The listing builds one solid part. Answer for the finished solid, in the listing's coordinates (mm). A direction names the side the tool comes from. Coordinates: 2 decimals unless noted, no trailing zeros. Loops run counter-clockwise (first coordinate to the right, second up) from the corner with the lowest first, then second, coordinate; pieces in that order, holes last. Notation, with made-up numbers: (48.25, -23.5) - (62.25, -23.5) arc R14 ccw to (62.25, -11.5) - close; hole circle Ø9 at (58, 71.5). An arc over 180 degrees is marked (long way). Write each question's results on one line, items separated by ' | '. Start each with the question number.
(1) Find section B-B on y = 30.5. Determine the outline of the cut face in (x, z).
(2) Determine the mould class of faces 6 (the flat face through (-66, 17, 1)), 7 (the flat face through (-1, 13, -47.5)), 8 (the cylindrical face through (-1.71, 6.75, -32.19)) for opening direction X: released by +X, released by -X, zero draft, split by the parting line, or undercut.
(3) Consider line 1 (X direction, y = 14, z = -22); line 2 (X direction, y = 4.05, z = 0) (3 decimals); line 3 (Z direction, x = 33.5, y = 25). Determine where each line is inside the solid, lowest interval first. Write a range as from..to.
(4) Find section D-D on x = -30. Determine the outline of the cut face in (y, z), then the cut area to 3 significant figures.
(5) Given pin 1 Ø3 at (x, z) = (0, -34.5) entering from +Y; pin 2 Ø3 at (x, z) = (49.5, 2) entering from +Y; pin 3 Ø5.5 at (x, z) = (26.625, 0) entering from +Y, each flat-ended and moving along its own axis, determine where each tip first touches the part or whether it passes through.
(6) For faces 1 (the cylindrical face through (63.5, 24.9, -10.7)), 2 (the flat face through (15, 15, 45)), 3 (the cylindrical face through (-33, 4, -1)), 4 (the flat face through (-10, 20, 28.363)), 5 (the cylindrical face through (-38.535, 1.521, -0.369)), determine the directions among +Z, -Z, +X, -X, +Y, -Y from which every point of the face is accessible in a straight line to the end or side of a thin tool.
(7) Find section C-C on z = -29. Determine the outline of the cut face in (x, y), then the cut area to 3 significant figures.
from build123d import *

# Parameters (mm, degrees)
SKETCH1_W           = 132
SKETCH1_H           = 95
BOSS_EXTRUDE1_DEPTH = 35
SKETCH2_W           = 122
SKETCH2_H           = 85
CUT_EXTRUDE1_DEPTH  = 30
SKETCH4_W           = 5
SKETCH4_H           = 85
BOSS_EXTRUDE2_DEPTH = 30
SKETCH5_R           = 2.5
SKETCH5_R_2         = 1.75
BOSS_EXTRUDE3_DEPTH = 2
FILLET1_R           = 1.5
SKETCH7_W           = 5
SKETCH7_H           = 10
CUT_EXTRUDE3_DEPTH  = 10
SKETCH8_R           = 1.75
SKETCH8_R_2         = 1.7
CUT_EXTRUDE4_DEPTH  = 10
SKETCH9_R           = 4
CUT_EXTRUDE6_DEPTH  = 2
SKETCH11_W          = 5.5
SKETCH11_H          = 12
SKETCH11_H_2        = 10
CUT_EXTRUDE7_DEPTH  = 10
SKETCH13_W          = 5.5
SKETCH13_H          = 10
CUT_EXTRUDE8_DEPTH  = 10
SKETCH14_W          = 5.5
SKETCH14_H          = 12
CUT_EXTRUDE9_DEPTH  = 10
SKETCH15_R          = 1.75
CUT_EXTRUDE10_DEPTH = 10


with BuildPart() as part:
    # Sketch1 → Boss-Extrude1 (new body)
    with BuildSketch(Plane(origin=(0, 0, 0), x_dir=(1, 0, 0), z_dir=(0, 1, 0))):
        Rectangle(SKETCH1_W, SKETCH1_H)
    extrude(amount=BOSS_EXTRUDE1_DEPTH)

    # Sketch2 → Cut-Extrude1 (cut)
    with BuildSketch(Plane(origin=(0, 35, 0), x_dir=(1, 0, 0), z_dir=(0, 1, 0))):
        Rectangle(SKETCH2_W, SKETCH2_H)
    extrude(amount=-CUT_EXTRUDE1_DEPTH, mode=Mode.SUBTRACT)

    # Sketch4 → Boss-Extrude2 (add, through all)
    with BuildSketch(Plane(origin=(0, 5, 0), x_dir=(1, 0, 0), z_dir=(0, 1, 0))):
        with Locations((-10.25, 0)):
            Rectangle(SKETCH4_W, SKETCH4_H)
    extrude(amount=BOSS_EXTRUDE2_DEPTH)

    # Sketch5 → Boss-Extrude3 (add)
    # profile 1 of 4: a face of its own
    with BuildSketch(Plane(origin=(0, 5, 0), x_dir=(1, 0, 0), z_dir=(0, 1, 0))):
        with Locations(Location((55.55, -35.5, 0), (0, 0, 270))):
            Circle(SKETCH5_R)
        with Locations(Location((55.55, -35.5, 0), (0, 0, 270))):
            Circle(SKETCH5_R_2, mode=Mode.SUBTRACT)
    # profile 2 of 4: a face of its own
    with BuildSketch(Plane(origin=(0, 5, 0), x_dir=(1, 0, 0), z_dir=(0, 1, 0))):
        with Locations(Location((-0.75, -35.5, 0), (0, 0, 270))):
            Circle(SKETCH5_R)
        with Locations(Location((-0.75, -35.5, 0), (0, 0, 270))):
            Circle(SKETCH5_R_2, mode=Mode.SUBTRACT)
    # profile 3 of 4: a face of its own
    with BuildSketch(Plane(origin=(0, 5, 0), x_dir=(1, 0, 0), z_dir=(0, 1, 0))):
        with Locations(Location((55.249999996, 34.49935714, 0), (0, 0, 270))):
            Circle(SKETCH5_R)
        with Locations(Location((55.249999996, 34.49935714, 0), (0, 0, 270))):
            Circle(SKETCH5_R_2, mode=Mode.SUBTRACT)
    # profile 4 of 4: a face of its own
    with BuildSketch(Plane(origin=(0, 5, 0), x_dir=(1, 0, 0), z_dir=(0, 1, 0))):
        with Locations(Location((-0.75, 34.5, 0), (0, 0, 270))):
            Circle(SKETCH5_R)
        with Locations(Location((-0.75, 34.5, 0), (0, 0, 270))):
            Circle(SKETCH5_R_2, mode=Mode.SUBTRACT)
    extrude(amount=BOSS_EXTRUDE3_DEPTH)

    # Fillet1
    fillet1_edges = [part.edges().sort_by_distance(p)[0] for p in [
        (55.55, 5, 33),
        (-0.75, 5, 33),
        (55.249999996, 5, -36.99935714),
        (-0.75, 5, -37),
    ]]
    fillet(fillet1_edges, radius=FILLET1_R)

    # Sketch7 → Cut-Extrude3 (cut)
    with BuildSketch(Plane(origin=(-7.75, 0, 0), x_dir=(0, 0, -1), z_dir=(1, 0, 0))):
        with Locations((-25.863290262, 20)):
            Rectangle(SKETCH7_W, SKETCH7_H)
    extrude(amount=-CUT_EXTRUDE3_DEPTH, mode=Mode.SUBTRACT)

    # Sketch8 → Cut-Extrude4 (cut)
    with BuildSketch(Plane(origin=(0, 5, 0), x_dir=(1, 0, 0), z_dir=(0, 1, 0))):
        with Locations(Location((26.625, 0, 0), (0, 0, 270))):
            Circle(SKETCH8_R)
        with Locations(Location((-36.875, 0, 0), (0, 0, 270))):
            Circle(SKETCH8_R_2)
    extrude(amount=-CUT_EXTRUDE4_DEPTH, mode=Mode.SUBTRACT)

    # Sketch9 → Cut-Extrude6 (cut)
    with BuildSketch(Plane(origin=(0, 5, 0), x_dir=(1, 0, 0), z_dir=(0, 1, 0))):
        with Locations(Location((26.625, 0, 0), (0, 0, 270))):
            Circle(SKETCH9_R)
        with Locations(Location((-36.875, 0, 0), (0, 0, 270))):
            Circle(SKETCH9_R)
    extrude(amount=-CUT_EXTRUDE6_DEPTH, mode=Mode.SUBTRACT)

    # Sketch11 → Cut-Extrude7 (cut)
    with BuildSketch(Plane.ZY.offset(-61)):
        with Locations((-1.95, 21)):
            Rectangle(SKETCH11_W, SKETCH11_H)
        with Locations((25.05, 20)):
            Rectangle(SKETCH11_W, SKETCH11_H_2)
        with BuildLine():
            Line((-14.75, 20.8), (-20.65, 20.8))
            ThreePointArc((-20.65, 20.8), (-24.7, 24.85), (-20.65, 28.9))
            Line((-20.65, 28.9), (-14.75, 28.9))
            ThreePointArc((-14.75, 28.9), (-10.7, 24.85), (-14.75, 20.8))
        make_face()
    extrude(amount=-CUT_EXTRUDE7_DEPTH, mode=Mode.SUBTRACT)

    # Sketch13 → Cut-Extrude8 (cut)
    with BuildSketch(Plane(origin=(0, 0, 42.5), x_dir=(-1, 0, 0), z_dir=(0, 0, -1))):
        with Locations((-15.42, 20)):
            Rectangle(SKETCH13_W, SKETCH13_H)
    extrude(amount=-CUT_EXTRUDE8_DEPTH, mode=Mode.SUBTRACT)

    # Sketch14 → Cut-Extrude9 (cut)
    with BuildSketch(Plane.XY.offset(-42.5)):
        with Locations((0.43, 21)):
            Rectangle(SKETCH14_W, SKETCH14_H)
    extrude(amount=-CUT_EXTRUDE9_DEPTH, mode=Mode.SUBTRACT)

    # Sketch15 → Cut-Extrude10 (cut)
    with BuildSketch(Plane(origin=(0, 35, 0), x_dir=(1, 0, 0), z_dir=(0, 1, 0))):
        with Locations(Location((-63.5, -3, 0), (0, 0, 270))):
            Circle(SKETCH15_R)
        with Locations(Location((63.5, -3, 0), (0, 0, 90))):
            Circle(SKETCH15_R)
    extrude(amount=-CUT_EXTRUDE10_DEPTH, mode=Mode.SUBTRACT)


solid = part.part
Values:
1) outline: (-66, -47.5) - (66, -47.5) - (66, 47.5) - (-66, 47.5) - close; hole circle Ø3.5 at (-63.5, 3); hole (-61, -42.5) - (-12.75, -42.5) - (-12.75, 42.5) - (-61, 42.5) - close; hole (-7.75, -42.5) - (61, -42.5) - (61, 42.5) - (-7.75, 42.5) - close; hole circle Ø3.5 at (63.5, 3)
2) face 6: released by -X | face 7: zero draft | face 8: undercut
3) line 1: x = -66..-61, -12.75..-7.75, 61..66 | line 2: x = -66..-40.875, -32.875..22.625, 30.625..66 | line 3: z = -47.5..-42.5, 42.5..47.5
4) outline: (0, -47.5) - (35, -47.5) - (35, -42.5) - (5, -42.5) - (5, 42.5) - (35, 42.5) - (35, 47.5) - (0, 47.5) - close | area: 775 mm²
5) pin 1: stops at y = 7 | pin 2: stops at y = 5 | pin 3: stops at y = 3
6) face 1: +X | face 2: +Z | face 3: +Y | face 4: none | face 5: +Y, -Y
7) outline: (-66, 0) - (66, 0) - (66, 35) - (61, 35) - (61, 5) - (-7.75, 5) - (-7.75, 35) - (-12.75, 35) - (-12.75, 5) - (-61, 5) - (-61, 35) - (-66, 35) - close | area: 1,110 mm²
